Input: part model. Units: mm. Frame: model coordinates. A direction names the side the tool comes from. Coordinates: 2 decimals unless noted, no trailing zeros. Loops run counter-clockwise (first coordinate to the right, second up) from the corner with the lowest first, then second, coordinate; pieces in that order, holes last.
(1) Section D-D, the plane z = 2.25. Return loops of the section in (x, y).
(2) Set-up query: faces 1 (the face through (14, -6, 1)), 2 (the face through (6, -6, 2)), 3 (the face through (10, -5, 3)), 4 (the face through (8.4, -2.93, 1.52)). Return all of +Z, -Z, +X, -X, +Y, -Y with unobstructed straight access to the full face (end or side cutting, diameter ignored); none if empty.
(3) Section A-A, the plane y = -3. Return loops of the section in (x, z).
(4) Section B-B, the plane x = 7.25. Return loops of the section in (y, z), then the cut area to 3 significant figures.
(5) Section C-C, the plane z = 10. Return loops of the section in (x, y), then the cut area to 3 significant figures.
(6) Mould query, pull axis X, two halves, no side actions, for faces 5 (the face through (20, 4, 9)), 6 (the face through (3, 21.29, 9)), 7 (the face through (5.804, 7.847, 10.185)). Classes: released by +X, released by -X, zero draft, split by the parting line, or undercut.
(7) Contact query for flat-ended pins moving along their axis: P1, Ø1, axis at y = 17.5, z = 11, coming from the +X side; P2, Ø2.5, axis at y = -7, z = 1, coming from the -X side; P3, Ø7.5, axis at x = 10, z = 10, coming from the +Y side; P4, Ø6.5, axis at x = 8.5, y = -5.5, coming from the +Z side. Output: stop coordinate, or through.
(8) Line query: L1, parallel to Z at x = 10, y = 7.75; L2, parallel to X at y = 8, z = 10; L3, parallel to Z at x = 12, y = -5.25. Output: solid intervals per line, ascending.
```python
from build123d import *

# Parameters (mm, degrees)
EXTRUDE_1_DEPTH     = 18
SKETCH_2_R          = 4.2
CUT_EXTRUDE_1_DEPTH = 28
EXTRUDE_2_DEPTH     = 8
SKETCH_4_R          = 1.6
CUT_EXTRUDE_2_DEPTH = 8
CHAMFER_1_SIZE      = 5
CHAMFER_2_SIZE      = 5


with BuildPart() as part:
    # 草图1 → 凸台-拉伸1 (new body)
    with BuildSketch(Plane.XY):
        with BuildLine():
            Line((0, 0), (20, 0))
            Line((20, 0), (20, 9.111319982))
            ThreePointArc((20, 9.111319982), (11.967350423, 14.437400737), (5.19, 21.29))
            Line((5.19, 21.29), (0, 21.29))
            Line((0, 21.29), (0, 0))
        make_face()
    extrude(amount=EXTRUDE_1_DEPTH)

    # 草图2 → 切除-拉伸1 (cut)
    with BuildSketch(Plane.XZ):
        with Locations((10, 10)):
            Circle(SKETCH_2_R)
    extrude(amount=-CUT_EXTRUDE_1_DEPTH, mode=Mode.SUBTRACT)

    # 草图3 → 凸台-拉伸2 (add)
    with BuildSketch(Plane.XZ):
        Polygon((10, 0), (14, 0), (14, 3), (6, 3), (6, 0), align=None)
    extrude(amount=EXTRUDE_2_DEPTH)

    # 草图4 → 切除-拉伸2 (cut)
    with BuildSketch(Plane.XY.offset(3)):
        with Locations((10, -3)):
            Circle(SKETCH_4_R)
    extrude(amount=-CUT_EXTRUDE_2_DEPTH, mode=Mode.SUBTRACT)

    # 倒角1
    chamfer_1_edges = [part.edges().sort_by_distance(p)[0] for p in [
        (6, 0, 1.5),
    ]]
    chamfer(chamfer_1_edges, length=CHAMFER_1_SIZE)

    # 倒角2
    chamfer_2_edges = [part.edges().sort_by_distance(p)[0] for p in [
        (14, 0, 1.5),
    ]]
    chamfer(chamfer_2_edges, length=CHAMFER_2_SIZE)


solid = part.part
```
Report:
1. outline: (0, 0) - (1, 0) - (6, -5) - (6, -8) - (14, -8) - (14, -5) - (19, 0) - (20, 0) - (20, 9.11) arc R47 cw to (5.19, 21.29) - (0, 21.29) - close; hole circle Ø3.2 at (10, -3)
2. face 1: +Z, -Z, +X, -Y
2. face 2: +Z, -Z, -X, -Y
2. face 3: +Z, +X, -X, -Y
2. face 4: +Z, -Z
3. outline: (4, 0) - (8.4, 0) - (8.4, 3) - (4, 3) - close; (11.6, 0) - (16, 0) - (16, 3) - (11.6, 3) - close
4. outline: (-8, 0) - (18.9, 0) - (18.9, 6.83) - (0, 6.83) - (0, 3) - (-8, 3) - close; (0, 13.17) - (18.9, 13.17) - (18.9, 18) - (0, 18) - close
4. area: 244 mm2
5. outline: (0, 0) - (5.8, 0) - (5.8, 20.55) arc R47 cw to (5.19, 21.29) - (0, 21.29) - close; (14.2, 0) - (20, 0) - (20, 9.11) arc R47 cw to (14.2, 12.71) - close
5. area: 186 mm2
6. face 5: released by +X
6. face 6: zero draft
6. face 7: undercut
7. P1: stops at x = 6.08
7. P2: stops at x = 6
7. P3: passes through
7. P4: stops at z = 3
8. L1: z = 0 to 5.8, 14.2 to 18
8. L2: x = 0 to 5.8, 14.2 to 20
8. L3: z = 0 to 3
